Design review of the part shown in the three views and the two pictorial views. Dimensions are in mm from the part's minimum x, y and z. A direction names the side the tool comes from. Give positions to 0.01 mm unless a question says otherwise; leave off trailing zeros. Write each loop counter-clockwise with the first axis right and the second up, starting at its lowest first coordinate (ties: lowest second). Pieces come first, ordered by that corner, then holes. Notation, with made-up numbers: M 45.25,41.25 L 64.25,41.25 A15 cw 64.25,68.25 Z; hole C 23.25,10 d6. An arc over 180 degrees is marked long. Write item = value, one per line.
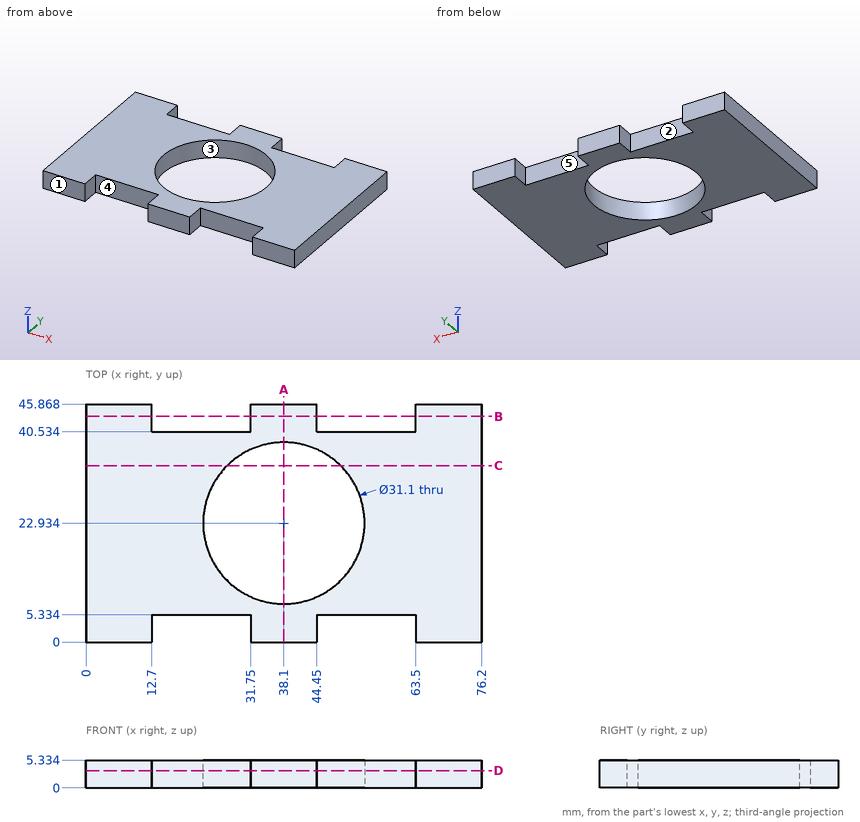
1. For line 1 along X through (y, z) = (3.5, 4.1); line 2 along Y through (x, z) = (38.1, 1.9); line 3 along X through (y, z) = (22.5, 1.95), list the stretches that pass through material, from the lowest coordinate up. Write a range as from..to.
Responses:
line_1 = 0..12.7, 31.75..44.45, 63.5..76.2
line_2 = 0..7.38, 38.48..45.87
line_3 = 0..22.56, 53.64..76.2
2. We need section B-B, the plane y = 43.5. Write out the cut boundary in (x, z), then the cut area to 3 significant figures.
Responses:
outline = M 0,0 L 12.7,0 L 12.7,5.33 L 0,5.33 Z; M 31.75,0 L 44.45,0 L 44.45,5.33 L 31.75,5.33 Z; M 63.5,0 L 76.2,0 L 76.2,5.33 L 63.5,5.33 Z
area = 203 mm2
3. We need section A-A, the plane x = 38.1. Write out the cut boundary in (y, z), then the cut area to 3 significant figures.
Responses:
outline = M 0,0 L 7.38,0 L 7.38,5.33 L 0,5.33 Z; M 38.48,0 L 45.87,0 L 45.87,5.33 L 38.48,5.33 Z
area = 78.8 mm2
4. Machinability: for the marked faces 3, 4 and 5, which of the approach directions +Z, -Z, +X, -X, +Y, -Y give a long, thin tool a straight path to every point of the face, cutting with its end or side? Answer none if there is none.
Responses:
face_3 = +Z, -Z
face_4 = +Z, -Z, -Y
face_5 = +Z, -Z, +Y
5. We need section C-C, the plane y = 34. Write out the cut boundary in (x, z).
Responses:
outline = M 0,0 L 27.18,0 L 27.18,5.33 L 0,5.33 Z; M 49.02,0 L 76.2,0 L 76.2,5.33 L 49.02,5.33 Z
6. The part is to be moulded in two halves that separate along X. For the marked faces 1 and 2, say which applies: +X half, -X half, draft (parallel to the pull), parting line (faces both ways), or undercut.
Responses:
face_1 = draft
face_2 = undercut
7. Insertion check: P1, Ø1, axis at x = 62, z = 2, coming from the -Y side. The pin has a flat end and moves straight along its axis. Give the tip position at first contact, or say it passes through.
Responses:
P1 = 5.33
8. We need section D-D, the plane z = 3.35. Write out the cut boundary in (x, y), then the cut area to 3 significant figures.
Responses:
outline = M 0,0 L 12.7,0 L 12.7,5.33 L 31.75,5.33 L 31.75,0 L 44.45,0 L 44.45,5.33 L 63.5,5.33 L 63.5,0 L 76.2,0 L 76.2,45.87 L 63.5,45.87 L 63.5,40.53 L 44.45,40.53 L 44.45,45.87 L 31.75,45.87 L 31.75,40.53 L 12.7,40.53 L 12.7,45.87 L 0,45.87 Z; hole C 38.1,22.93 d31.1
area = 2,330 mm2
